from build123d import *

# Parameters (mm, degrees)
BOSS_EXTRUDE1_DEPTH = 10


with BuildPart() as part:
    # Sketch1 → Boss-Extrude1 (new body)
    with BuildSketch(Plane(origin=(0, 0, 0), x_dir=(1, 0, 0), z_dir=(0, 1, 0))):
        with BuildLine():
            Line((0, 120), (0, 60))
            Line((0, 60), (12.294200791, 60))
            ThreePointArc((12.294200791, 60), (17.5, 65.205799209), (22.705799209, 60))
            Line((22.705799209, 60), (35, 60))
            Line((35, 60), (35, 120))
            Line((35, 120), (0, 120))
        make_face()
        with BuildLine():
            Line((0, 60), (0, 0))
            Line((0, 0), (35, 0))
            Line((35, 0), (35, 60))
            Line((35, 60), (22.705799209, 60))
            ThreePointArc((22.705799209, 60), (17.5, 54.794200791), (12.294200791, 60))
            Line((12.294200791, 60), (0, 60))
        make_face()
    extrude(amount=BOSS_EXTRUDE1_DEPTH)


solid = part.part
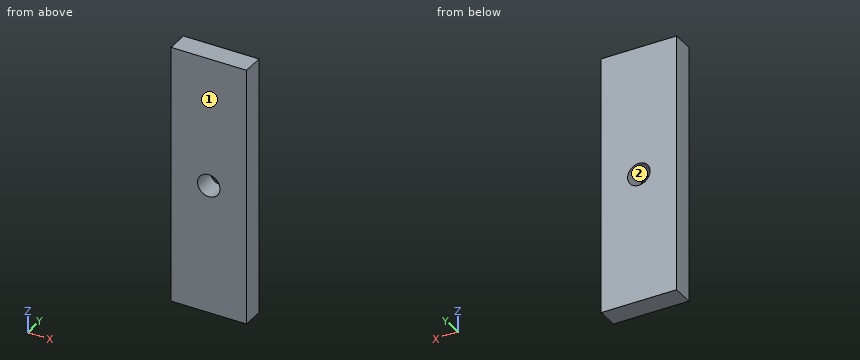
Read the model definition and answer for the solid it produces. Units are mm, in the model's axes. Face numbers are marked on the shaded views. Give positions to 0.01 mm unless a question says otherwise; leave off trailing zeros. Write each loop counter-clockwise with the first axis right and the second up, starting at its lowest first coordinate (ties: lowest second). Pieces come first, ordered by that corner, then holes. Notation, with made-up numbers: M 28,-15 L 65,-15 A34 ccw 65,24 Z; hole C 17.25,53 d4. An arc over 180 degrees is marked long. One line per item, written item: value. Start each with the question number.
(1) Find section C-C (y = 5.75). Determine the outline of the cut face in (x, z), plus the area to 3 significant figures.
(2) Find section A-A (x = 17.5). Determine the outline of the cut face in (y, z).
(3) Find section B-B (z = -60). Determine the outline of the cut face in (x, y).
(4) Determine the mould class of the marked faces 1 and 2 for opening direction X: pulls with the +X half, pulls with the -X half, needs draft (parallel to the pull), parting line crosses it, or undercut.
(5) Find the intervals of material crossed by line 1 (Z direction, x = 17.5, y = 5.5); line 2 (X direction, y = 2, z = -62); line 3 (Z direction, x = 22, y = 5.5), in increasing order.
Results below:
1. outline: M 0,-120 L 35,-120 L 35,0 L 0,0 Z; hole C 17.5,-60 d10.41
1. area: 4,110 mm^2
2. outline: M 0,-120 L 10,-120 L 10,-65.21 L 0,-65.21 Z; M 0,-54.79 L 10,-54.79 L 10,0 L 0,0 Z
3. outline: M 0,0 L 12.29,0 L 12.29,10 L 0,10 Z; M 22.71,0 L 35,0 L 35,10 L 22.71,10 Z
4. face 1: needs draft
4. face 2: undercut
5. line 1: z = -120 to -65.21, -54.79 to 0
5. line 2: x = 0 to 12.69, 22.31 to 35
5. line 3: z = -120 to -62.62, -57.38 to 0
